from build123d import *

# Parameters (mm, degrees)
SKETCH_1_R          = 7.5
SKETCH_1_W          = 22
SKETCH_1_H          = 30
EXTRUDE_1_DEPTH     = 52
SKETCH_2_W          = 30
SKETCH_2_H          = 35
CUT_EXTRUDE_1_DEPTH = 108.721864076
SKETCH_3_W          = 46
SKETCH_3_H          = 44
CUT_EXTRUDE_2_DEPTH = 108.721864076
SKETCH_4_W          = 52
SKETCH_4_H          = 50
EXTRUDE_2_DEPTH     = 5
SKETCH_5_R          = 10
CUT_EXTRUDE_3_DEPTH = 112.485425056


with BuildPart() as part:
    # ｽｹｯﾁ1 → ﾎﾞｽ - 押し出し1 (new body)
    with BuildSketch(Plane.XY):
        with BuildLine():
            Line((0, 0), (55, 0))
            ThreePointArc((55, 0), (80, -25), (55, -50))
            Line((55, -50), (0, -50))
            Line((0, -50), (0, 0))
        make_face()
        with Locations(Location((55, -25, 0), (0, 0, 180))):
            Circle(SKETCH_1_R, mode=Mode.SUBTRACT)
        with Locations((21, -25)):
            Rectangle(SKETCH_1_W, SKETCH_1_H, mode=Mode.SUBTRACT)
    extrude(amount=EXTRUDE_1_DEPTH)

    # ｽｹｯﾁ2 → ｶｯﾄ - 押し出し1 (cut, through all)
    with BuildSketch(Plane(origin=(0, 0, 0), x_dir=(1, 0, 0), z_dir=(0, 1, 0))):
        with Locations((30, -26)):
            Rectangle(SKETCH_2_W, SKETCH_2_H)
    extrude(amount=-CUT_EXTRUDE_1_DEPTH, mode=Mode.SUBTRACT)

    # ｽｹｯﾁ3 → ｶｯﾄ - 押し出し2 (cut, through all)
    with BuildSketch(Plane.ZY):
        with Locations((26, -25)):
            Rectangle(SKETCH_3_W, SKETCH_3_H)
    extrude(amount=-CUT_EXTRUDE_2_DEPTH, mode=Mode.SUBTRACT)

    # ｽｹｯﾁ4 → ﾎﾞｽ - 押し出し2 (add)
    with BuildSketch(Plane.ZY):
        with Locations((26, -25)):
            Rectangle(SKETCH_4_W, SKETCH_4_H)
    extrude(amount=EXTRUDE_2_DEPTH)

    # ｽｹｯﾁ5 → ｶｯﾄ - 押し出し3 (cut, through all)
    with BuildSketch(Plane.ZY.offset(5)):
        with Locations(Location((26, -25, 0), (0, 0, 270))):
            Circle(SKETCH_5_R)
    extrude(amount=-CUT_EXTRUDE_3_DEPTH, mode=Mode.SUBTRACT)


solid = part.part
Geometry check sheet. Reference: the model listing, model coordinates, mm. A direction names the side the tool comes from. Give positions to 0.01 mm unless a question says otherwise; leave off trailing zeros. Order: outer loops, then holes, each group sorted by start corner. A loop starts at its lowest first (then second) coordinate and runs counter-clockwise, first axis right, second up. Notation, with made-up numbers: M 66.5,36 L 71.5,36 A30 cw 71.5,60 Z; hole C 26.5,35 d6. An arc over 180 degrees is marked long. Use a Markdown table: item, result.
Item 1: Section check C-C (y = -25). Record the cut outline in (x, z), and give its area (3 significant figures).
Answers follow:
| item | result |
|---|---|
| outline | M -5,0 L 10,0 L 10,3 L 0,3 L 0,16 L -5,16 Z; M -5,36 L 0,36 L 0,49 L 10,49 L 10,52 L -5,52 Z; M 32,0 L 47.5,0 L 47.5,3 L 32,3 Z; M 32,49 L 47.5,49 L 47.5,52 L 32,52 Z; M 62.5,0 L 80,0 L 80,3 L 62.5,3 Z; M 62.5,49 L 80,49 L 80,52 L 62.5,52 Z |
| area | 418 mm2 |
Item 2: Section check A-A (z = 26). Record the cut outline in (x, y), and give its area (3 significant figures).
Answers follow:
| item | result |
|---|---|
| outline | M -5,-50 L 15,-50 L 15,-47 L 0,-47 L 0,-35 L -5,-35 Z; M -5,-15 L 0,-15 L 0,-3 L 15,-3 L 15,0 L -5,0 Z; M 45,-50 L 55,-50 A25 ccw 66.87,-47 L 45,-47 Z; M 45,-3 L 66.87,-3 A25 ccw 55,0 L 45,0 Z |
| area | 348 mm2 |
Item 3: Depth check by flat-ended pin: P1, Ø3, axis at y = -44, z = 43, coming from the +X side; P2, Ø3.5, axis at y = -49, z = 22.5, coming from the +X side. Enter the tip coordinate at first touch or a pass-through.
Answers follow:
| item | result |
|---|---|
| P1 | stops at x = 0 |
| P2 | stops at x = 66.4 |
Item 4: Material ranges on line 1 along X through (y, z) = (-25, 51); line 2 along Z through (x, y) = (36.5, -36); line 3 along Z through (x, y) = (-1.8, -25), recorded low to high.
Answers follow:
| item | result |
|---|---|
| line 1 | x = -5 to 10, 32 to 47.5, 62.5 to 80 |
| line 2 | z = 0 to 3, 49 to 52 |
| line 3 | z = 0 to 16, 36 to 52 |
Item 5: Draft check along X on faces 1 (the flat face through (-5, -14, 26)), 2 (the flat face through (30, -1, 43.5)), 3 (the flat face through (48, -47, 26)). Enter one of: +X half, -X half, draft (parallel to the pull), parting line (faces both ways), or undercut.
Answers follow:
| item | result |
|---|---|
| face 1 | -X half |
| face 2 | undercut |
| face 3 | draft |
Item 6: Section check D-D (y = -33.5). Record the cut outline in (x, z).
Answers follow:
| item | result |
|---|---|
| outline | M -5,0 L 10,0 L 10,3 L 0,3 L 0,20.73 L -5,20.73 Z; M -5,31.27 L 0,31.27 L 0,49 L 10,49 L 10,52 L -5,52 Z; M 32,0 L 78.51,0 L 78.51,3 L 32,3 Z; M 32,49 L 78.51,49 L 78.51,52 L 32,52 Z |
Item 7: Tool access check on faces 4 (the flat face through (30, -48, 43.5)), 5 (the flat face through (21, -10, 1)), 6 (the flat face through (39, -25, 3)). Record the directions out of +Z, -Z, +X, -X, +Y, -Y that give a thin tool (end or side, any length) a straight path to the whole face; none if there is none.
Answers follow:
| item | result |
|---|---|
| face 4 | +Y, -Y |
| face 5 | +Z, -Z |
| face 6 | +X |
Item 8: Section check B-B (x = 42). Record the cut outline in (y, z).
Answers follow:
| item | result |
|---|---|
| outline | M -50,0 L 0,0 L 0,8.5 L -3,8.5 L -3,3 L -47,3 L -47,8.5 L -50,8.5 Z; M -50,43.5 L -47,43.5 L -47,49 L -3,49 L -3,43.5 L 0,43.5 L 0,52 L -50,52 Z |
